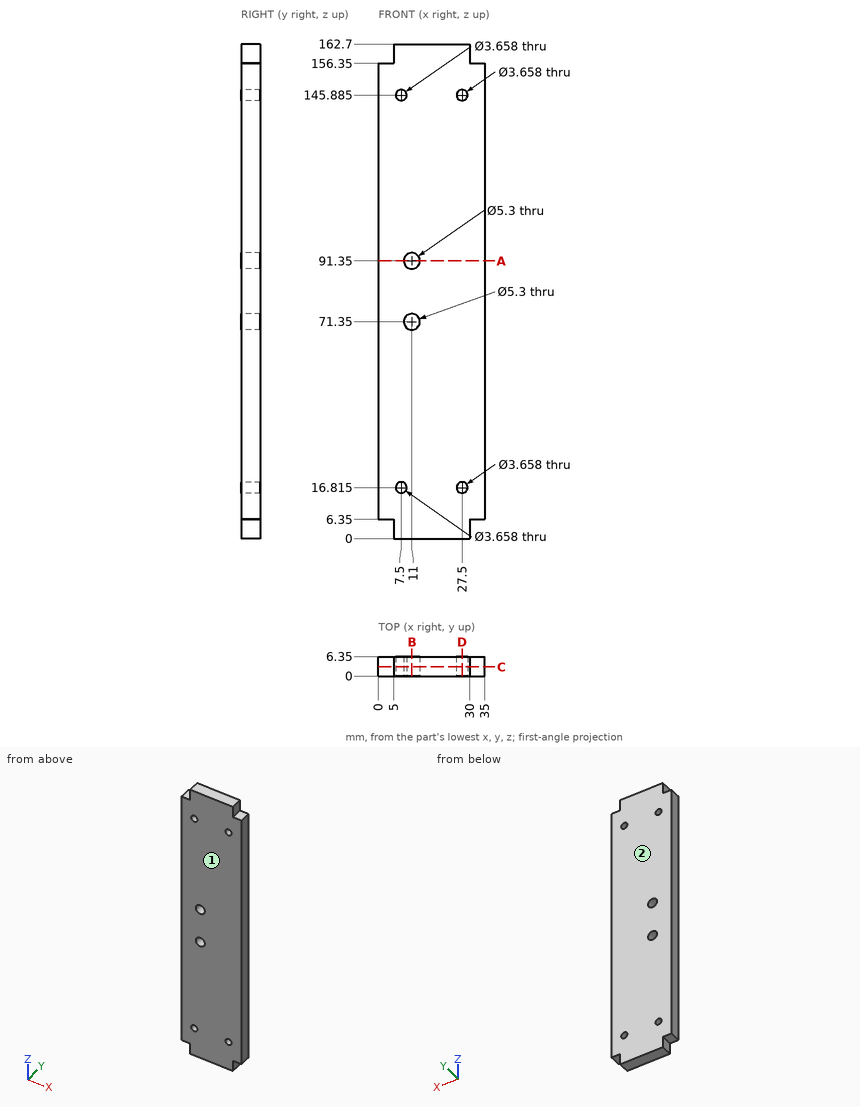
Input: dimensioned drawing with shaded views. Units: mm. Origin: part minimum x, y, z. Coordinates: 2 decimals unless noted, no trailing zeros. Order: outer loops, then holes, each group sorted by start corner. A loop starts at its lowest first (then second) coordinate and runs counter-clockwise, first axis right, second up. Notation, with made-up numbers: (28.5, 42) - (50.5, 42) arc R23 cw to (50.5, 58) - close; hole circle Ø9 at (31.25, -20.5). An arc over 180 degrees is marked (long way). Return JSON: item names as keys, results as strings. Group by question number.
1. Material intervals for line 1 along Z through (x, y) = (26.5, 2) (1 decimal); line 2 along Z through (x, y) = (12, 2.75) (1 decimal); line 3 along X through (y, z) = (1.5, 91.35), sorted ascending. Write a range as [from, to].
2. Cut plane B-B (x = 11). Output: boundary loops of the cut face in (y, z).
3. Pull-direction query (Y, two-part tool) for the marked faces 1 and 2; classes: pulls with the +Y half, pulls with the -Y half, needs draft (parallel to the pull), parting line crosses it, or undercut.
4. Pin query (flat end, axial travel): pin 1 (3 mm diameter, centred on y = 1.5, z = 4.5, fed in from -X); pin 2 (3 mm diameter, centred on y = 2.5, z = 158.5, fed in from +X); pin 3 (1.5 mm diameter, centred on x = 33, y = 3.5, fed in from +Z). Return the tip coordinate at first contact, or that it passes through.
5. Cut plane C-C (y = 3). Count the separate pieces of the cut face and the enclosed holes in it, plus the area to 3 significant figures.
6. Cut plane D-D (x = 27.5). Output: boundary loops of the cut face in (y, z).
7. Cut plane A-A (z = 91.35). Output: boundary loops of the cut face in (x, y), plus the area to 3 significant figures.
Resolved:
{
 "1": {"line 1": "z = [0, 15.3], [18.3, 144.4], [147.4, 162.7]", "line 2": "z = [0, 68.9], [73.8, 88.9], [93.8, 162.7]", "line 3": "x = [0, 8.35], [13.65, 35]"},
 "2": {"outline": "(0, 0) - (6.35, 0) - (6.35, 68.7) - (0, 68.7) - close; (0, 74) - (6.35, 74) - (6.35, 88.7) - (0, 88.7) - close; (0, 94) - (6.35, 94) - (6.35, 162.7) - (0, 162.7) - close"},
 "3": {"face 1": "pulls with the -Y half", "face 2": "pulls with the +Y half"},
 "4": {"pin 1": "stops at x = 5", "pin 2": "stops at x = 30", "pin 3": "stops at z = 156.35"},
 "5": {"separate pieces": "1", "enclosed holes": "6", "area": "5,480 mm²"},
 "6": {"outline": "(0, 0) - (6.35, 0) - (6.35, 14.99) - (0, 14.99) - close; (0, 18.64) - (6.35, 18.64) - (6.35, 144.06) - (0, 144.06) - close; (0, 147.71) - (6.35, 147.71) - (6.35, 162.7) - (0, 162.7) - close"},
 "7": {"outline": "(0, 0) - (8.35, 0) - (8.35, 6.35) - (0, 6.35) - close; (13.65, 0) - (35, 0) - (35, 6.35) - (13.65, 6.35) - close", "area": "189 mm²"}
}
